Model file for the job. Use its own axes, mm. A direction names the side the tool comes from. Coordinates: 2 decimals unless noted, no trailing zeros. Order: outer loops, then holes, each group sorted by start corner. A loop starts at its lowest first (then second) coordinate and runs counter-clockwise, first axis right, second up. Notation, with made-up numbers: M 84.5,19.25 L 119.5,19.25 A22 cw 119.5,44.25 Z; hole C 2,30.25 d9. An arc over 180 degrees is marked long. Return JSON: item names as keys, results as strings.
```python
from build123d import *

# Parameters (mm, degrees)
SKETCH1_R           = 40
BOSS_EXTRUDE1_DEPTH = 3
CUT_EXTRUDE1_DEPTH  = 3


with BuildPart() as part:
    # Sketch1 → Boss-Extrude1 (new body)
    with BuildSketch(Plane.XY):
        Circle(SKETCH1_R)
    extrude(amount=BOSS_EXTRUDE1_DEPTH)

    # Sketch2 → Cut-Extrude1 (cut)
    with BuildSketch(Plane(origin=(0, 0, 0), x_dir=(-1, 0, 0), z_dir=(0, 0, -1))):
        Polygon((0, -35), (4.5, -35), (4.5, -32), (-4.5, -32), (-4.5, -35), align=None)
    extrude(amount=-CUT_EXTRUDE1_DEPTH, mode=Mode.SUBTRACT)


solid = part.part
```
Item 1: 3-axis set-ups, long thin cutter, end or side, ignore diameter. For faces 1 (the flat face through (4.5, -33, 1)), 2 (the flat face through (-1, 1, 0)): which of +Z, -Z, +X, -X, +Y, -Y reach the whole face in a straight line?
Check result:
{"face 1": "+Z, -Z", "face 2": "-Z, +X, -X, +Y, -Y"}
Item 2: Saw through at D-D (y = 26.5). Write the cut outline in (x, z), and give its area (3 significant figures).
Check result:
{"outline": "M -29.96,0 L 29.96,0 L 29.96,3 L -29.96,3 Z", "area": "180 mm2"}
Item 3: Wall check: line 1 (X direction, y = -33, z = 1.5); line 2 (Y direction, x = 3, z = 0.45); line 3 (Y direction, x = 15, z = 2.8). Give the ranges that are in metal, low to high.
Check result:
{"line 1": "x = -22.61 to -4.5, 4.5 to 22.61", "line 2": "y = -39.89 to -35, -32 to 39.89", "line 3": "y = -37.08 to 37.08"}
Item 4: Drop flat-ended pins along their axis: pin 1 Ø1 at (y, z) = (-26, 0.5) entering from -X; pin 2 Ø1.5 at (x, z) = (-0.5, 1) entering from -Y; pin 3 Ø1.5 at (y, z) = (-33.5, 1) entering from +X. Give the stop position or say it passes through.
Check result:
{"pin 1": "stops at x = -30.82", "pin 2": "stops at y = -40", "pin 3": "stops at x = 22.97"}
Item 5: Saw through at C-C (x = 22.5). Write the cut outline in (y, z).
Check result:
{"outline": "M -33.07,0 L 33.07,0 L 33.07,3 L -33.07,3 Z"}
Item 6: Saw through at B-B (z = 1.8). Write the cut outline in (x, y), and give its area (3 significant figures).
Check result:
{"outline": "C 0,0 d80; hole M -4.5,-35 L 4.5,-35 L 4.5,-32 L -4.5,-32 Z", "area": "5,000 mm2"}
Item 7: Pull direction X, two halves, no side cores. Call faces 3 (the flat face through (-1, 1, 3)), 4 (the cylindrical face through (-8.67, -39.05, 1.48)), 5 (the flat face through (0, -35, 1)): +X half, -X half, draft (parallel to the pull), parting line (faces both ways), or undercut.
Check result:
{"face 3": "draft", "face 4": "parting line", "face 5": "undercut"}
Item 8: Saw through at A-A (x = 0). Write the cut outline in (y, z).
Check result:
{"outline": "M -40,0 L -35,0 L -35,3 L -40,3 Z; M -32,0 L 40,0 L 40,3 L -32,3 Z"}
